from build123d import *

# Parameters (mm, degrees)
F1_DEPTH = 5.08
F2_DEPTH = 25.4
F4_DEPTH = 50.8


with BuildPart() as f1:
    # F0 (on Top) → F1 (new body)
    with BuildSketch(Plane.XY):
        Polygon((-127, 127), (-127, -127), (127, -127), (127, 127), (0, 127), align=None)
    extrude(amount=F1_DEPTH)

    # F0 (on Top) → F2 (join)
    with BuildSketch(Plane.XY):
        Polygon((-127, -152.4), (-127, -127), (-127, 127), (-127, 279.4), (-152.4, 279.4), (-152.4, -127), (-152.4, -152.4), align=None)
        Polygon((127, 127), (127, -127), (127, -152.4), (152.4, -152.4), (152.4, -127), (152.4, 279.4), (127, 279.4), align=None)
    extrude(amount=F2_DEPTH)

    # F3 (on face) → F4 (join)
    with BuildSketch(Plane.YZ.offset(152.4)):
        Polygon((168.895449, 31.75), (-168.895449, 31.75), (-168.895449, -31.75), (-91.065334, -97.057221), (244.749885, -97.057221), (322.58, -31.75), (322.58, 31.75), align=None)
    extrude(amount=F4_DEPTH)


solid = f1.part
Source: CAD feature listing. Evaluate the final solid. Frame: model axes, mm. A direction names the side the tool comes from. Give positions to 0.01 mm unless a question says otherwise; leave off trailing zeros. Write each loop counter-clockwise with the first axis right and the second up, starting at its lowest first coordinate (ties: lowest second). Pieces come first, ordered by that corner, then holes. Notation, with made-up numbers: (46.25, -28.75) - (53.25, -28.75) arc R13 cw to (53.25, -23.75) - close; hole circle Ø7 at (66.5, 78). An arc over 180 degrees is marked (long way). Write item = value, one per line. Start each with the question number.
Q1. Draft query along X for faces 1 (the flat face through (140, -152.4, 13)), 2 (the flat face through (-152.4, 67, 13)), 3 (the flat face through (203.2, 73, -32)), 4 (the flat face through (-127, 60, 13)). Return one class per face: +X half, -X half, draft (parallel to the pull), parting line (faces both ways), or undercut.
Q2. Cut plane D-D, the plane x = -38.5. Return loops of the section in (y, z), then the cut area to 3 significant figures.
Q3. Cut plane C-C, the plane y = 13.5. Return loops of the section in (x, z).
Q4. Pin query (flat end, axial travel): pin 1 Ø8 at (y, z) = (225, -84) entering from -X; pin 2 Ø12.5 at (x, z) = (-143.5, 17) entering from +Y; pin 3 Ø5.5 at (x, z) = (-26, 3.5) entering from +Y. Return the tip coordinate at first contact, or that it passes through.
Q5. Cut plane B-B, the plane y = 185.5. Return loops of the section in (x, z), then the cut area to 3 significant figures.
Q6. Material intervals for probe 1 along X at (y, z) = (126, 22); probe 2 along X at (y, z) = (63.5, -69.5); probe 3 along Z at (x, y) = (-88.5, -46), sorted ascending.
Q7. Cut plane A-A, the plane z = 11. Return loops of the section in (x, y), then the cut area to 3 significant figures.
Q8. Reachability of faces 5 (the flat face through (-2, 2, 5.08)), 6 (the flat face through (140, 279.4, 13)), 7 (the flat face through (140, 67, 25.4)), 8 (the flat face through (-140, -152.4, 13)) from +Z, -Z, +X, -X, +Y, -Y: full face, straight path, thin tool, end or side. Return the list, or none.
Computed values:
q1.face_1 = draft
q1.face_2 = -X half
q1.face_3 = +X half
q1.face_4 = undercut
q2.outline = (-127, 0) - (127, 0) - (127, 5.08) - (-127, 5.08) - close
q2.area = 1,290 mm²
q3.outline = (-152.4, 0) - (152.4, 0) - (152.4, -97.06) - (203.2, -97.06) - (203.2, 31.75) - (152.4, 31.75) - (152.4, 25.4) - (127, 25.4) - (127, 5.08) - (-127, 5.08) - (-127, 25.4) - (-152.4, 25.4) - close
q4.pin_1 = 152.4
q4.pin_2 = 279.4
q4.pin_3 = 127
q5.outline = (-152.4, 0) - (-127, 0) - (-127, 25.4) - (-152.4, 25.4) - close; (127, 0) - (152.4, 0) - (152.4, -97.06) - (203.2, -97.06) - (203.2, 31.75) - (152.4, 31.75) - (152.4, 25.4) - (127, 25.4) - close
q5.area = 7,830 mm²
q6.probe_1 = -152.4 to -127, 127 to 203.2
q6.probe_2 = 152.4 to 203.2
q6.probe_3 = 0 to 5.08
q7.outline = (-152.4, -152.4) - (-127, -152.4) - (-127, 279.4) - (-152.4, 279.4) - close; (127, -152.4) - (152.4, -152.4) - (152.4, -168.9) - (203.2, -168.9) - (203.2, 322.58) - (152.4, 322.58) - (152.4, 279.4) - (127, 279.4) - close
q7.area = 46,900 mm²
q8.face_5 = +Z, +Y, -Y
q8.face_6 = +Z, -Z, -X, +Y
q8.face_7 = +Z, -X, +Y, -Y
q8.face_8 = +Z, -Z, -X, -Y
